Part print with two shaded views. Sizes in mm from the minimum x, y, z corner. A direction names the side the tool comes from. Coordinates: 2 decimals unless noted, no trailing zeros. Order: outer loops, then holes, each group sorted by start corner. A loop starts at its lowest first (then second) coordinate and runs counter-clockwise, first axis right, second up. Notation, with made-up numbers: (-20.5, -37) - (8.5, -37) arc R20 ccw to (8.5, -3) - close; hole circle Ø6 at (87, -25.5). An arc over 180 degrees is marked (long way). Return JSON: item names as keys, results as strings.
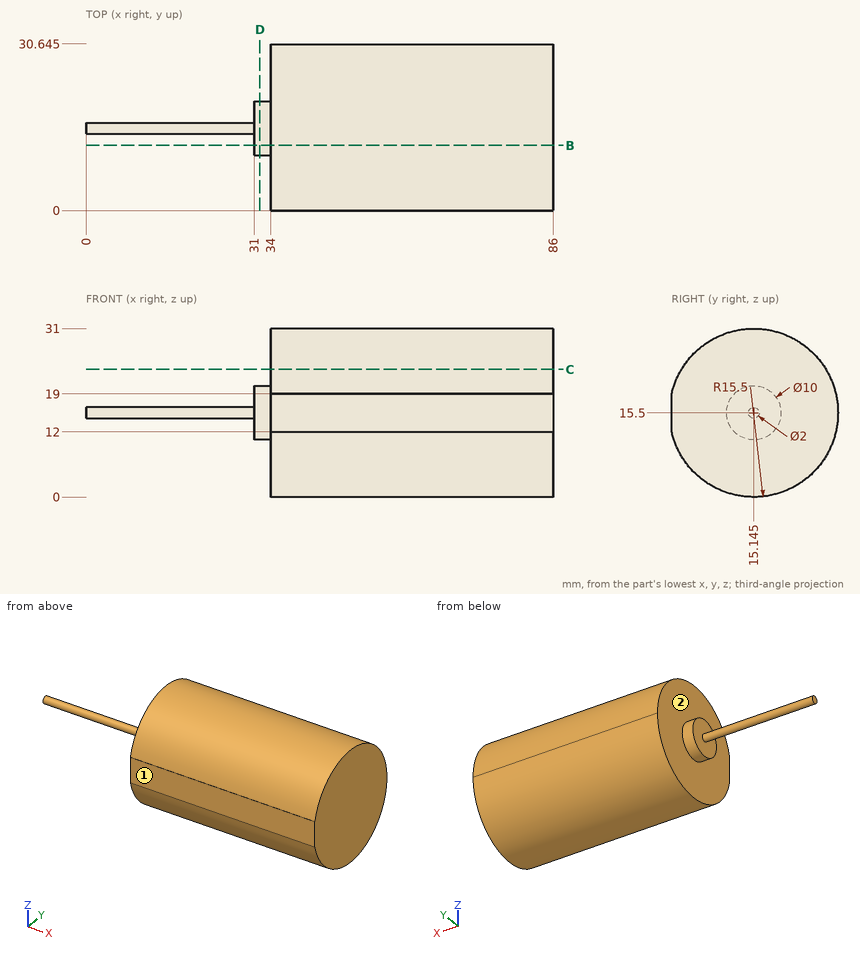
Item 1: Band-saw the part on B-B, the plane y = 12. List the corners of the cut face in (x, z), then the cut area to 3 significant figures.
Findings below:
{"outline": "(31, 11.61) - (34, 11.61) - (34, 0.32) - (86, 0.32) - (86, 30.68) - (34, 30.68) - (34, 19.39) - (31, 19.39) - close", "area": "1,600 mm²"}
Item 2: Band-saw the part on C-C, the plane z = 23.5. List the corners of the cut face in (x, y), then the cut area to 3 significant figures.
Findings below:
{"outline": "(34, 1.87) - (86, 1.87) - (86, 28.42) - (34, 28.42) - close", "area": "1,380 mm²"}
Item 3: Which spindle directions (+Z, -Z, +X, -X, +Y, -Y) get a long thin tool onto all of the face, cutting with end or side? Do the marked faces 1 and 2. Say none if no direction does.
Findings below:
{"face 1": "+Z, -Z, +X, -X, -Y", "face 2": "-X"}
Item 4: Band-saw the part on D-D, the plane x = 32. List the corners of the cut face in (y, z) (1 decimal).
Findings below:
{"outline": "circle Ø10 at (15.1, 15.5)"}
Item 5: Wall check: L1, parallel to X at y = 24, z = 20.5; L2, parallel to X at y = 15.5, z = 18.5; L3, parallel to Z at x = 67.5, y = 15.5. Give the ranges that are in metal, low to high. Write a range as [from, to].
Findings below:
{"L1": "x = [34, 86]", "L2": "x = [31, 86]", "L3": "z = [0, 31]"}
Item 6: Drop flat-ended pins along their axis: P1, Ø12, axis at x = 14, y = 15, coming from the -Z side; P2, Ø1, axis at y = 9, z = 13, coming from the -X side; P3, Ø8, axis at y = 22, z = 16.5, coming from the -X side. Give the stop position or say it passes through.
Findings below:
{"P1": "stops at z = 14.5", "P2": "stops at x = 34", "P3": "stops at x = 31"}
